Drawing for the job (mm, zero at the part's lowest x, y, z). A direction names the side the tool comes from. Round coordinates to 2 decimals unless told otherwise and drop trailing zeros. Loops run counter-clockwise (first coordinate to the right, second up) from the corner with the lowest first, then second, coordinate; pieces in that order, holes last. Notation, with made-up numbers: (-23.5, -15) - (2.5, -15) arc R14 cw to (2.5, -9) - close; hole circle Ø5 at (72, 75). An arc over 180 degrees is marked (long way). Put each result on its own line as item: value.
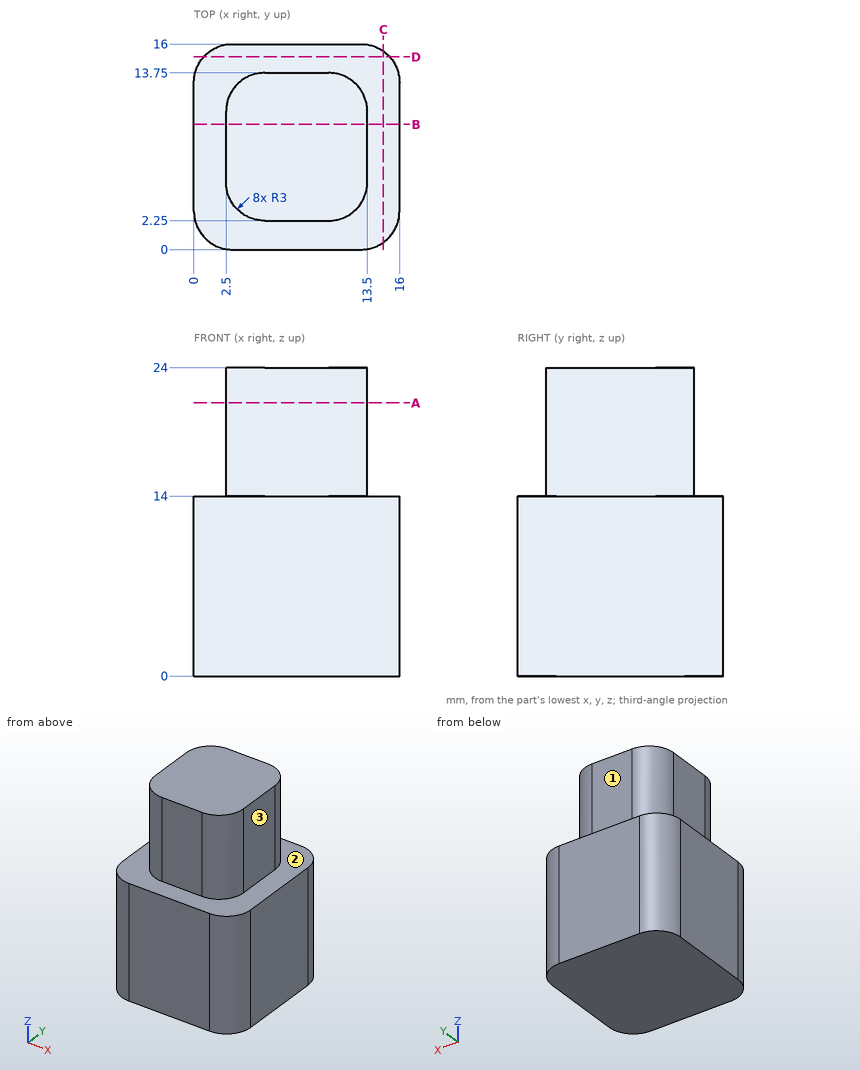
1. Tool access for the marked faces 1, 2 and 3: list every direction of +Z, -Z, +X, -X, +Y, -Y with a clear straight run to the whole face (end or side of a thin tool).
A:
face 1: +Z, +X, -X, +Y
face 2: +Z
face 3: +Z, +X, +Y, -Y
2. Probe line 1 along Z through (x, y) = (13, 3.5); line 2 along X through (y, z) = (5.25, 17.5); line 3 along Y through (x, z) = (7.25, 15.25). List the from-to ranges inside material, lowest first. Write a range as [from, to].
A:
line 1: z = [0, 14]
line 2: x = [2.5, 13.5]
line 3: y = [2.25, 13.75]
3. Band-saw the part on A-A (z = 21.25). List the corners of the cut face in (x, y).
A:
outline: (2.5, 5.25) arc R3 ccw to (5.5, 2.25) - (10.5, 2.25) arc R3 ccw to (13.5, 5.25) - (13.5, 10.75) arc R3 ccw to (10.5, 13.75) - (5.5, 13.75) arc R3 ccw to (2.5, 10.75) - close
4. Pin check, flat tips, straight feed: P1, Ø3, axis at y = 6.5, z = 18, coming from the -X side; P2, Ø6, axis at y = 9, z = 19.5, coming from the +X side; P3, Ø2, axis at y = 1.5, z = 11.5, coming from the +X side. Stop position of each tip, or through.
A:
P1: stops at x = 2.5
P2: stops at x = 13.5
P3: stops at x = 15.96
5. Band-saw the part on B-B (y = 9.75). List the corners of the cut face in (x, z), plus the area to 3 significant figures.
A:
outline: (0, 0) - (16, 0) - (16, 14) - (13.5, 14) - (13.5, 24) - (2.5, 24) - (2.5, 14) - (0, 14) - close
area: 334 mm²
6. Band-saw the part on D-D (y = 15). List the corners of the cut face in (x, z).
A:
outline: (0.76, 0) - (15.24, 0) - (15.24, 14) - (0.76, 14) - close
7. Band-saw the part on C-C (x = 14.75). List the corners of the cut face in (y, z).
A:
outline: (0.56, 0) - (15.44, 0) - (15.44, 14) - (0.56, 14) - close
